Geometry: final body of the model. Coordinates: model frame, mm. Round coordinates to 2 decimals unless told otherwise and drop trailing zeros. Write each loop counter-clockwise with the first axis right and the second up, starting at its lowest first coordinate (ties: lowest second). Pieces come first, ordered by that corner, then holes. Notation, with made-up numbers: (59, 74.5) -> (104, 74.5) arc R16 ccw to (104, 82.5) -> close; hole circle Ø6 at (4, 31). An arc over 180 degrees is marked (long way). One line per item, written item: value. Start each with the question number.
from build123d import *

# Parameters (mm, degrees)
SKETCH1_W           = 88.9
SKETCH1_H           = 76.2
BOSS_EXTRUDE1_DEPTH = 1.6
SKETCH2_R           = 2.15
CUT_EXTRUDE1_DEPTH  = 2.6
SKETCH4_R           = 1.905
CUT_EXTRUDE2_DEPTH  = 2.6
FILLET1_R           = 6.35


with BuildPart() as part:
    # Sketch1 → Boss-Extrude1 (new body)
    with BuildSketch(Plane.XY):
        with Locations((28.959521177, 30.063142475)):
            Rectangle(SKETCH1_W, SKETCH1_H)
    extrude(amount=BOSS_EXTRUDE1_DEPTH)

    # Sketch2 → Cut-Extrude1 (cut, through all)
    with BuildSketch(Plane(origin=(0, 0, 0), x_dir=(-1, 0, 0), z_dir=(0, 0, -1))):
        with Locations((-23.890706089, 38.789996981)):
            Circle(SKETCH2_R)
        with Locations((3.822106833, 38.789996981)):
            Circle(SKETCH2_R)
        with Locations((-10.034299628, 62.789996981)):
            Circle(SKETCH2_R)
    extrude(amount=-CUT_EXTRUDE1_DEPTH, mode=Mode.SUBTRACT)

    # Sketch4 → Cut-Extrude2 (cut, through all)
    with BuildSketch(Plane(origin=(0, 0, 0), x_dir=(-1, 0, 0), z_dir=(0, 0, -1))):
        with Locations((10.410478823, 63.083142475)):
            Circle(SKETCH4_R)
        with Locations((-68.329521177, 63.083142475)):
            Circle(SKETCH4_R)
        with Locations((-68.329521177, -2.956857525)):
            Circle(SKETCH4_R)
        with Locations((10.410478823, -2.956857525)):
            Circle(SKETCH4_R)
    extrude(amount=-CUT_EXTRUDE2_DEPTH, mode=Mode.SUBTRACT)

    # Fillet1
    fillet1_edges = [part.edges().sort_by_distance(p)[0] for p in [
        (-15.490478823, 68.163142475, 0.8),
        (73.409521177, 68.163142475, 0.8),
        (73.409521177, -8.036857525, 0.8),
        (-15.490478823, -8.036857525, 0.8),
    ]]
    fillet(fillet1_edges, radius=FILLET1_R)


solid = part.part
(1) Line query: probe 1 along X at (y, z) = (-2, 1.05); probe 2 along Y at (x, z) = (67, 0.6); probe 3 along X at (y, z) = (61, 0.25). Output: solid intervals per line, ascending.
(2) Section query B-B (z = 0.4). Output: boundary loops of the cut face in (x, y) (3 decimals), and give its area (3 significant figures).
(3) Section query A-A (x = 68.5). Output: boundary loops of the cut face in (y, z), and give its area (3 significant figures).
(4) Pull-direction query (X, two-part tool) for faces 1 (the face through (71.5, 66.35, 0.81)), 2 (the face through (-13.68, -6.127, 0.811)), 3 (the face through (-3.36, 36.69, 0.79)); classes: pulls with the +X half, pulls with the -X half, needs draft (parallel to the pull), parting line crosses it, or undercut.
Results list:
1. probe 1: x = -15.48 to -12.06, -8.76 to 66.68, 69.98 to 73.4
1. probe 2: y = -8.04 to -4.32, -1.59 to 61.72, 64.45 to 68.16
1. probe 3: x = -15.49 to 8.84, 11.23 to 73.41
2. outline: (-15.49, -1.687) arc R6.35 ccw to (-9.14, -8.037) -> (67.06, -8.037) arc R6.35 ccw to (73.41, -1.687) -> (73.41, 61.813) arc R6.35 ccw to (67.06, 68.163) -> (-9.14, 68.163) arc R6.35 ccw to (-15.49, 61.813) -> close; hole circle Ø3.81 at (-10.41, -2.957); hole circle Ø3.81 at (-10.41, 63.083); hole circle Ø4.3 at (-3.822, 38.79); hole circle Ø4.3 at (10.034, 62.79); hole circle Ø4.3 at (23.891, 38.79); hole circle Ø3.81 at (68.33, -2.957); hole circle Ø3.81 at (68.33, 63.083)
2. area: 6,650 mm^2
3. outline: (-7.87, 0) -> (-4.85, 0) -> (-4.85, 1.6) -> (-7.87, 1.6) -> close; (-1.06, 0) -> (61.19, 0) -> (61.19, 1.6) -> (-1.06, 1.6) -> close; (64.98, 0) -> (68, 0) -> (68, 1.6) -> (64.98, 1.6) -> close
3. area: 109 mm^2
4. face 1: pulls with the +X half
4. face 2: pulls with the -X half
4. face 3: undercut
